Answer from the drawing. Dimensions are ordinates in mm from the lowest x, y and z of the part. A direction names the side the tool comes from. Round coordinates to 2 decimals unless told otherwise and drop trailing zeros. Order: outer loops, then holes, each group sorted by start corner. A loop starts at its lowest first (then second) coordinate and runs counter-clockwise, first axis right, second up. Notation, with made-up numbers: (41, 76) -> (79, 76) arc R13 ccw to (79, 82) -> close; hole circle Ø11 at (30, 65). An arc over 180 degrees is marked (long way). Use a Markdown table: item, result. Add a question column.
1. For the marked faces 1 and 2, determine the directions among +Z, -Z, +X, -X, +Y, -Y from which every point of the face is accessible in a straight line to the end or side of a thin tool.
2. Consider L1, parallel to X at y = 11.05, z = 124.46; L2, parallel to X at y = 11.9, z = 67.31 (1 decimal); L3, parallel to Y at x = 86, z = 228 (1 decimal). Determine where each line is inside the solid, lowest interval first. Write a range as [from, to].
3. Section A-A, the plane x = 151 is taken. Give the vertices of the cut face in (y, z) (1 decimal).
4. Given pin 1 (5 mm diameter, centred on x = 223.45, z = 67.31, fed in from -Y) (3 decimals); pin 2 (4 mm diameter, centred on x = 223.45, z = 181.61, fed in from -Y); pin 3 (3 mm diameter, centred on y = 6.5, z = 160, fed in from +X) (1 decimal); pin 4 (4 mm diameter, centred on x = 166, y = 8.5, fed in from -Z), each flat-ended and moving along its own axis, determine where each tip first touches the part or whether it passes through.
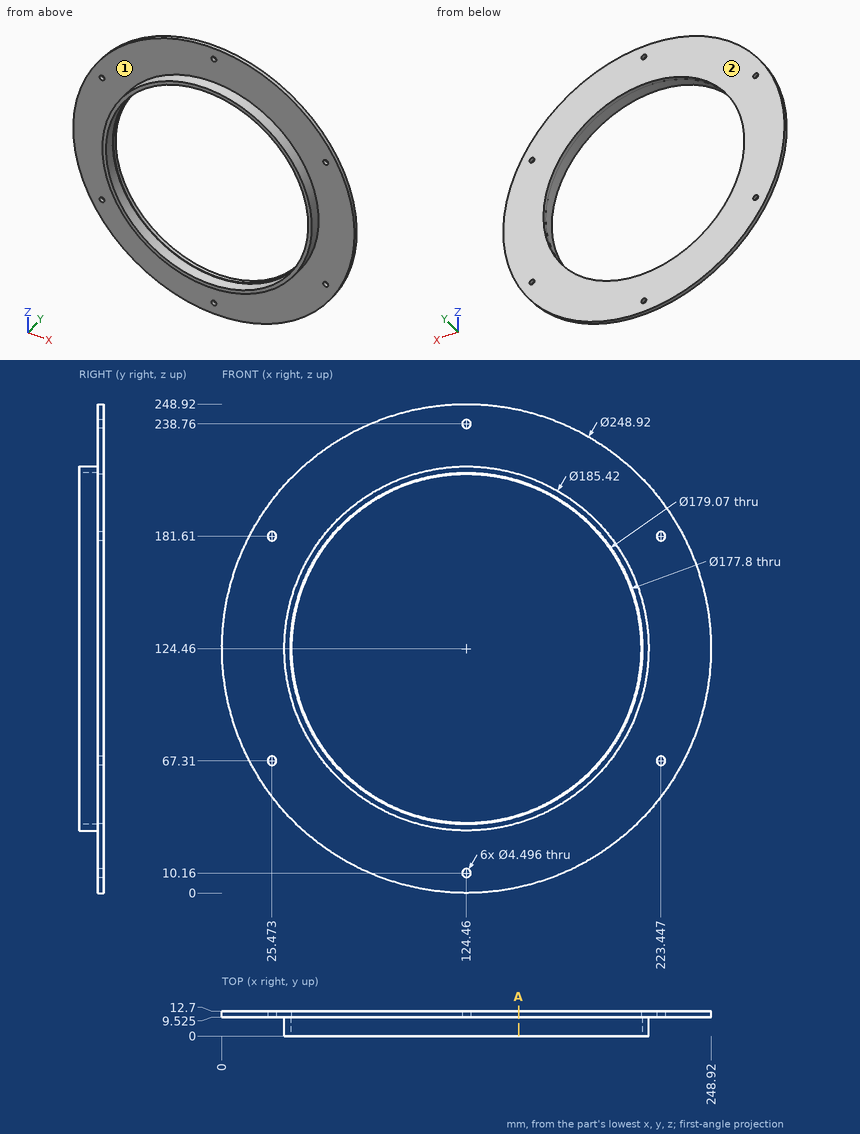
Verdict:
| question | item | result |
|---|---|---|
| 1 | face 1 | -Y |
| 1 | face 2 | +Z, -Z, +X, -X, +Y |
| 2 | L1 | x = [0, 35.56], [213.36, 248.92] |
| 2 | L2 | x = [13.9, 23.2], [27.7, 56.4], [192.6, 221.2], [225.7, 235] |
| 2 | L3 | y = [9.5, 12.7] |
| 3 | outline | (0, 35.6) -> (9.5, 35.6) -> (9.5, 2.9) -> (12.7, 2.9) -> (12.7, 39.6) -> (9.5, 39.6) -> (9.5, 38.9) -> (0, 38.9) -> close; (0, 210) -> (9.5, 210) -> (9.5, 209.3) -> (12.7, 209.3) -> (12.7, 246.1) -> (9.5, 246.1) -> (9.5, 213.3) -> (0, 213.3) -> close |
| 4 | pin 1 | stops at y = 9.525 |
| 4 | pin 2 | passes through |
| 4 | pin 3 | stops at x = 210.7 |
| 4 | pin 4 | stops at z = 6.54 |
